Can you work these out from the model? Positions are in its coordinate system, mm. A direction names the side the tool comes from. Give positions to 0.01 mm unless a question says otherwise; leave off trailing zeros. Order: outer loops, then holes, each group sorted by start corner. A loop starts at its lowest first (then second) coordinate and runs counter-clockwise, first axis right, second up. Notation, with made-up numbers: M 89,-4.5 L 102,-4.5 A20 ccw 102,23.5 Z; hole C -11,27.25 d8. An arc over 180 degrees is marked long. One line per question, with ' | ' between items. Start each with the question number.
1) If we section it at D-D, the plane z = -30: Please give me the cut outline in (x, y), plus the area to 3 significant figures.
2) If we section it at B-B, the plane z = -23: Please give me the cut outline in (x, y), plus the area to 3 significant figures.
3) Please list where these lines run through material, in increasing order: line 1 along X through (y, z) = (4, -30); line 2 along X through (y, z) = (2.5, -36); line 3 along Z through (x, y) = (45.5, 2). Write a range as [from, to].
4) If we section it at C-C, the plane y = 4.5: Please give me the cut outline in (x, z), plus the area to 3 significant figures.
5) If we section it at A-A, the plane x = 15.5: Please give me the cut outline in (y, z).
6) For faces 1 (the flat face through (25, 5, 0)), 2 (the flat face through (40.7, 5, -20)), which set-ups out of +Z, -Z, +X, -X, +Y, -Y let a thin tool reach every point of the face, with its end or its side?
7) Thinking about a two-plate mould opening in X: for faces 3 (the cylindrical face through (50.1, 5.07, -40.43)), 4 (the flat face through (25, 5, -5.5)), 5 (the flat face through (25, 5, -41)), 6 (the cylindrical face through (10.9, 5.07, -34.64)), which applies, +X half, -X half, draft (parallel to the pull), parting line (faces both ways), or undercut?
```python
from build123d import *

# Parameters (mm, degrees)
SKETCH_2_W      = 50.7
SKETCH_2_H      = 41
SKETCH_2_R      = 1.6
SKETCH_2_R_2    = 2.15
SKETCH_2_R_3    = 1.65
SKETCH_2_W_2    = 30.7
SKETCH_2_H_2    = 30
EXTRUDE_1_DEPTH = 10
FILLET_1_R      = 2
FILLET_2_R      = 3


with BuildPart() as part:
    # ｽｹｯﾁ2 → ﾎﾞｽ - 押し出し1 (new body)
    with BuildSketch(Plane(origin=(0, 0, 0), x_dir=(1, 0, 0), z_dir=(0, 1, 0))):
        with Locations((25.35, 20.5)):
            Rectangle(SKETCH_2_W, SKETCH_2_H)
        with Locations(Location((4, 36, 0), (0, 0, 270))):
            Circle(SKETCH_2_R, mode=Mode.SUBTRACT)
        with Locations(Location((3.25, 30, 0), (0, 0, 270))):
            Circle(SKETCH_2_R_2, mode=Mode.SUBTRACT)
        with Locations(Location((3.25, 5, 0), (0, 0, 270))):
            Circle(SKETCH_2_R_2, mode=Mode.SUBTRACT)
        with Locations(Location((45.7, 33.5, 0), (0, 0, 270))):
            Circle(SKETCH_2_R_3, mode=Mode.SUBTRACT)
        with Locations(Location((45.7, 7.5, 0), (0, 0, 90))):
            Circle(SKETCH_2_R_3, mode=Mode.SUBTRACT)
        with Locations((25.35, 20.5)):
            Rectangle(SKETCH_2_W_2, SKETCH_2_H_2, mode=Mode.SUBTRACT)
    extrude(amount=EXTRUDE_1_DEPTH)

    # ﾌｨﾚｯﾄ1
    fillet_1_edges = [part.edges().sort_by_distance(p)[0] for p in [
        (0, 5, -41),
        (50.7, 5, -41),
        (50.7, 5, 0),
        (0, 5, 0),
    ]]
    fillet(fillet_1_edges, radius=FILLET_1_R)

    # ﾌｨﾚｯﾄ2
    fillet_2_edges = [part.edges().sort_by_distance(p)[0] for p in [
        (40.7, 5, -5.5),
        (40.7, 5, -35.5),
        (10, 5, -35.5),
        (10, 5, -5.5),
    ]]
    fillet(fillet_2_edges, radius=FILLET_2_R)


solid = part.part
```
Results found:
1) outline: M 0,0 L 1.1,0 L 1.1,10 L 0,10 Z; M 5.4,0 L 10,0 L 10,10 L 5.4,10 Z; M 40.7,0 L 50.7,0 L 50.7,10 L 40.7,10 Z | area: 157 mm²
2) outline: M 0,0 L 10,0 L 10,10 L 0,10 Z; M 40.7,0 L 50.7,0 L 50.7,10 L 40.7,10 Z | area: 200 mm²
3) line 1: x = [0, 1.1], [5.4, 10], [40.7, 50.7] | line 2: x = [0, 2.4], [5.6, 50.7] | line 3: z = [-41, -35.14], [-31.86, -9.14], [-5.86, 0]
4) outline: M 0,-39 A2 ccw 2,-41 L 48.7,-41 A2 ccw 50.7,-39 L 50.7,-2 A2 ccw 48.7,0 L 2,0 A2 ccw 0,-2 Z; hole C 3.25,-30 d4.3; hole C 3.25,-5 d4.3; hole C 4,-36 d3.2; hole M 10,-32.5 A3 ccw 13,-35.5 L 37.7,-35.5 A3 ccw 40.7,-32.5 L 40.7,-8.5 A3 ccw 37.7,-5.5 L 13,-5.5 A3 ccw 10,-8.5 Z; hole C 45.7,-33.5 d3.3; hole C 45.7,-7.5 d3.3 | area: 1,110 mm²
5) outline: M 0,-41 L 10,-41 L 10,-35.5 L 0,-35.5 Z; M 0,-5.5 L 10,-5.5 L 10,0 L 0,0 Z
6) face 1: +Z, +X, -X, +Y, -Y | face 2: +Y, -Y
7) face 3: +X half | face 4: undercut | face 5: draft | face 6: undercut
